Geometry: final body of the model. Coordinates: model frame, mm. Give positions to 0.01 mm unless a question says otherwise; leave off trailing zeros. Write each loop counter-clockwise with the first axis right and the second up, starting at its lowest first coordinate (ties: lowest second). Pieces come first, ordered by that corner, then holes. Notation, with made-up numbers: (85.5, -31.75) -> (111.5, -31.75) arc R18 ccw to (111.5, 3.25) -> close; hole circle Ø1 at (16, 60.5). An arc over 180 degrees is marked (long way). Answer as a JSON object with one key per item and string values.
from build123d import *

# Parameters (mm, degrees)
SKETCH2_W           = 40
SKETCH2_H           = 70
BOSS_EXTRUDE1_DEPTH = 5
FILLET1_R           = 15
CUT_EXTRUDE1_DEPTH  = 6
SKETCH4_R           = 0.75
CUT_EXTRUDE2_DEPTH  = 6


with BuildPart() as part:
    # Sketch2 → Boss-Extrude1 (new body)
    with BuildSketch(Plane(origin=(0, 0, 0), x_dir=(1, 0, 0), z_dir=(0, 1, 0))):
        with BuildLine():
            Line((-20, -35), (20, -35))
            ThreePointArc((20, -35), (0, -49.312603136), (-20, -35))
        make_face()
        Rectangle(SKETCH2_W, SKETCH2_H)
        with BuildLine():
            ThreePointArc((-20, 35), (0, 49.305454963), (20, 35))
            Line((20, 35), (-20, 35))
        make_face()
    extrude(amount=BOSS_EXTRUDE1_DEPTH)

    # Fillet1
    fillet1_edges = [part.edges().sort_by_distance(p)[0] for p in [
        (-20, 2.5, 35),
        (-20, 2.5, -35),
        (20, 2.5, -35),
        (20, 2.5, 35),
    ]]
    fillet(fillet1_edges, radius=FILLET1_R)

    # Sketch3 → Cut-Extrude1 (cut, through all)
    with BuildSketch(Plane.XZ):
        Polygon((0, 49.312603136), (1.823748233, 49.312603136), (1.823748233, 24.312603136), (-2.176251767, 24.312603136), (-2.176251767, 49.312603136), align=None)
    extrude(amount=-CUT_EXTRUDE1_DEPTH, mode=Mode.SUBTRACT)

    # Sketch4 → Cut-Extrude2 (cut, through all)
    with BuildSketch(Plane.XZ):
        with Locations((0, -43.172046648)):
            Circle(SKETCH4_R)
        with Locations((0, -11.172046648)):
            Circle(SKETCH4_R)
    extrude(amount=-CUT_EXTRUDE2_DEPTH, mode=Mode.SUBTRACT)


solid = part.part
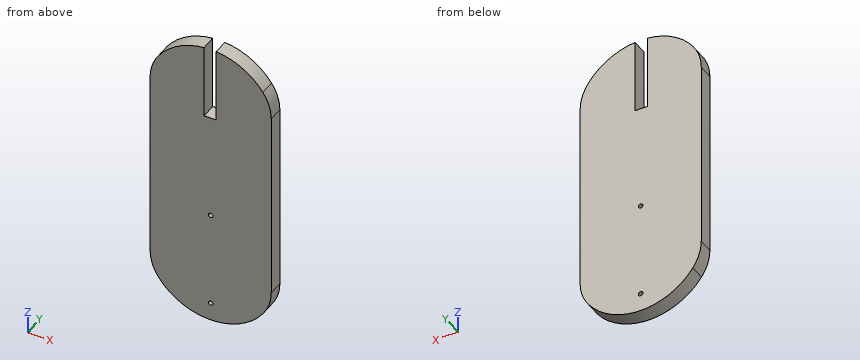
Q1. Cut plane B-B (x = 11). Return the cut outline in (y, z), and give its area (3 significant figures).
Values:
{"outline": "(0, -46.22) -> (5, -46.22) -> (5, 46.22) -> (0, 46.22) -> close", "area": "462 mm²"}
Q2. Cut plane C-C (x = 15). Return the cut outline in (y, z).
Values:
{"outline": "(0, -43.06) -> (5, -43.06) -> (5, 43.06) -> (0, 43.06) -> close"}
Q3. Cut plane A-A (y = 1.3). Return the cut outline in (x, z).
Values:
{"outline": "(-20, -31.72) arc R15 ccw to (-17.23, -40.41) arc R21.13 ccw to (17.23, -40.41) arc R15 ccw to (20, -31.72) -> (20, 31.73) arc R15 ccw to (17.23, 40.41) arc R21.13 ccw to (1.82, 49.23) -> (1.82, 24.31) -> (-2.18, 24.31) -> (-2.18, 49.2) arc R21.13 ccw to (-17.23, 40.41) arc R15 ccw to (-20, 31.73) -> close; hole circle Ø1.5 at (0, -43.17); hole circle Ø1.5 at (0, -11.17)"}
Q4. First-contact query: P1, Ø2, axis at x = -4.5, y = 3.5, coming from the -Z side; P2, Ø2.5, axis at y = 2.5, z = 42, coming from the +X side; P3, Ø6, axis at x = 9, z = -23.5, coming from the -Y side; P4, Ø1.5, axis at y = 1.5, z = 35, coming from the -X side. Flat tips, straight axial feed; report the tip coordinate or a pass-through.
Values:
{"P1": "z = -49.01", "P2": "x = 16.99", "P3": "y = 0", "P4": "x = -19.79"}
Q5. Material intervals for L1, parallel to X at y = 1.4, z = 25; L2, parallel to X at y = 1.3, z = 44; L3, parallel to X at y = 1.8, z = -40, sorted ascending. Write a range as from..to.
Values:
{"L1": "-20..-2.18, 1.82..20", "L2": "-14.01..-2.18, 1.82..14.01", "L3": "-17.51..17.51"}
